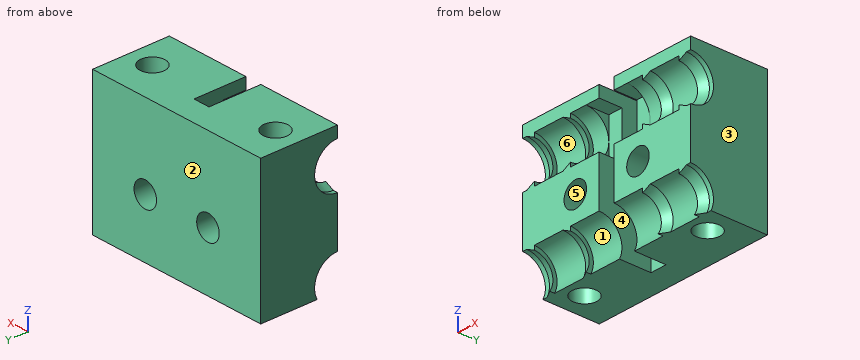
from build123d import *

# Parameters (mm, degrees)
REVOLVE1_ANGLE           = 180
BOSS_EXTRUDE1_DEPTH      = 9.25
BOSS_EXTRUDE1_DEPTH_BACK = 9.25
BOSS_EXTRUDE2_START      = 3.5
BOSS_EXTRUDE2_DEPTH      = 5.75
BOSS_EXTRUDE3_START      = -3.5
BOSS_EXTRUDE3_DEPTH      = 5.75
SKETCH14_W               = 2.5
SKETCH14_H               = 5
CUT_EXTRUDE10_DEPTH      = 13.7
SKETCH13_W               = 5.5
SKETCH13_H               = 2.75
CUT_EXTRUDE9_DEPTH       = 1.75
SKETCH15_W               = 12.7
SKETCH15_H               = 8
CUT_EXTRUDE11_DEPTH      = 6
SKETCH16_W               = 5.122625222
SKETCH16_H               = 5
CUT_EXTRUDE12_DEPTH      = 13.7
SKETCH22_W               = 2.5
SKETCH22_H               = 5
CUT_EXTRUDE17_DEPTH      = 17.877374778
SKETCH17_W               = 10.2
SKETCH17_H               = 16.877374778
BOSS_EXTRUDE4_DEPTH      = 4.25
SKETCH18_R               = 1.5
CUT_EXTRUDE13_DEPTH      = 10.25
SKETCH19_R               = 1.5
CUT_EXTRUDE14_DEPTH      = 6
SKETCH20_R               = 1.5
CUT_EXTRUDE16_DEPTH      = 17.877374778
SKETCH23_W               = 16.877374778
SKETCH23_H               = 3
BOSS_EXTRUDE5_DEPTH      = 1


with BuildPart() as part:
    # Sketch6 → Revolve1 (revolve)
    with BuildSketch(Plane(origin=(0, 0, 0), x_dir=(1, 0, 0), z_dir=(0, 1, 0))):
        Polygon((0, 5), (0, 2.75), (3.81, 2.75), (3.81, 2.242), (4.826, 2.75), (8.636, 2.75), (8.636, 2.242), (9.652, 2.75), (12.7, 2.75), (12.7, 5), align=None)
    revolve(axis=Axis((0, 0, 0), (1, 0, 0)), revolution_arc=REVOLVE1_ANGLE)

    # Sketch9 → Boss-Extrude1 (add, two sides)
    with BuildSketch(Plane.XY) as boss_extrude1_sk:
        Polygon((0, 3.25), (0, 5), (12.7, 5), (12.7, 2.75), align=None)
    extrude(amount=BOSS_EXTRUDE1_DEPTH)
    extrude(boss_extrude1_sk.sketch, amount=-BOSS_EXTRUDE1_DEPTH_BACK)

    # Sketch9_3 → Boss-Extrude2 (add)
    with BuildSketch(Plane.XY.offset(BOSS_EXTRUDE2_START)):
        Polygon((0, 3.25), (12.7, 2.75), (12.7, 0), (0, 0), align=None)
    extrude(amount=BOSS_EXTRUDE2_DEPTH)

    # Sketch9_4 → Boss-Extrude3 (add)
    with BuildSketch(Plane.XY.offset(BOSS_EXTRUDE3_START)):
        Polygon((0, 3.25), (12.7, 2.75), (12.7, 0), (0, 0), align=None)
    extrude(amount=-BOSS_EXTRUDE3_DEPTH)

    # Sketch14 → Cut-Extrude10 (cut, through all)
    with BuildSketch(Plane.ZY):
        with Locations((-8, 2.5)):
            Rectangle(SKETCH14_W, SKETCH14_H)
    extrude(amount=-CUT_EXTRUDE10_DEPTH, mode=Mode.SUBTRACT)

    # Mirror4: part across plane


with BuildPart() as part_1:
    add(part.part)
    add(part.part.mirror(Plane.XY.offset(-5.75)))

    # Sketch13 → Cut-Extrude9 (cut)
    with BuildSketch(Plane.ZY):
        with Locations((0, 1.375)):
            Rectangle(SKETCH13_W, SKETCH13_H)
    extrude(amount=-CUT_EXTRUDE9_DEPTH, mode=Mode.SUBTRACT)

    # Sketch15 → Cut-Extrude11 (cut, through all)
    with BuildSketch(Plane(origin=(0, 5, 0), x_dir=(1, 0, 0), z_dir=(0, 1, 0))):
        with Locations((6.35, 16.75)):
            Rectangle(SKETCH15_W, SKETCH15_H)
    extrude(amount=-CUT_EXTRUDE11_DEPTH, mode=Mode.SUBTRACT)

    # Sketch16 → Cut-Extrude12 (cut, through all)
    with BuildSketch(Plane.ZY):
        with Locations((6.688687389, 2.5)):
            Rectangle(SKETCH16_W, SKETCH16_H)
    extrude(amount=-CUT_EXTRUDE12_DEPTH, mode=Mode.SUBTRACT)

    # Sketch22 → Cut-Extrude17 (cut, through all)
    with BuildSketch(Plane.XY.offset(4.127374778)):
        with Locations((11.45, 2.5)):
            Rectangle(SKETCH22_W, SKETCH22_H)
    extrude(amount=-CUT_EXTRUDE17_DEPTH, mode=Mode.SUBTRACT)


with BuildPart() as body_2:
    # Mirror8: mirrored copy
    add(part_1.part.mirror(Plane.XY.offset(5.397374778)))

    # Sketch19 → Cut-Extrude14 (cut, through all)
    with BuildSketch(Plane(origin=(0, 5, 0), x_dir=(1, 0, 0), z_dir=(0, 1, 0))):
        with Locations((3.175, -16.573374778)):
            Circle(SKETCH19_R)
    extrude(amount=-CUT_EXTRUDE14_DEPTH, mode=Mode.SUBTRACT)


with BuildPart() as part_2:
    add(part_1.part)

    # Sketch17 → Boss-Extrude4 (add)
    with BuildSketch(Plane(origin=(0, 5, 0), x_dir=(1, 0, 0), z_dir=(0, 1, 0))):
        with Locations((5.1, 4.311312611)):
            Rectangle(SKETCH17_W, SKETCH17_H)
    extrude(amount=BOSS_EXTRUDE4_DEPTH)

    # Sketch18 → Cut-Extrude13 (cut, through all)
    with BuildSketch(Plane(origin=(0, 9.25, 0), x_dir=(1, 0, 0), z_dir=(0, 1, 0))):
        with Locations((3.175, 5.778625222)):
            Circle(SKETCH18_R)
    extrude(amount=-CUT_EXTRUDE13_DEPTH, mode=Mode.SUBTRACT)

    # Sketch20 → Cut-Extrude16 (cut, through all)
    with BuildSketch(Plane.XY.offset(4.127374778)):
        with Locations((7.2, 4.75)):
            Circle(SKETCH20_R)
    extrude(amount=-CUT_EXTRUDE16_DEPTH, mode=Mode.SUBTRACT)

    # Sketch23 → Boss-Extrude5 (add)
    with BuildSketch(Plane.ZY):
        with Locations((-4.311312611, 7.75)):
            Rectangle(SKETCH23_W, SKETCH23_H)
    extrude(amount=BOSS_EXTRUDE5_DEPTH)


with BuildPart() as body_3:
    # Mirror9: mirrored copy
    add(part_2.part.mirror(Plane.ZY.offset(1)))

    # Combine1: union part
    add(part_2.part)


solid = body_3.part
The listing builds one solid part. Answer for the finished solid, in the listing's coordinates (mm). Face numbers are marked on the shaded views. A direction names the side the tool comes from. Round coordinates to 2 decimals unless told otherwise and drop trailing zeros. Write each loop counter-clockwise with the first axis right and the second up, starting at its lowest first coordinate (ties: lowest second). Pieces come first, ordered by that corner, then holes. Notation, with made-up numbers: (-26.75, 16.25) - (-3.75, 16.25) arc R18 cw to (-3.75, 26.25) - close; hole circle Ø2 at (-16, 55.5). An arc over 180 degrees is marked (long way). Use a Markdown table: item, result. Add a question column.
1. The part is cut by section A-A (y = 4.75). Write down the section's boundary in (x, z) (3 decimals).
2. A tool of negligible diameter and unlimited length cuts with its end or side. For the marked faces 4, 5 and 6, from which of +Z, -Z, +X, -X, +Y, -Y can it reach the whole face along a straight path? Write none if from no direction.
3. The part is cut by section B-B (z = -3). Write down the section's boundary in (x, y).
4. For a pull along X with two mould halves and no side action, classify the marked faces 1, 2 and 3 as +X half, -X half, draft (parallel to the pull), parting line (faces both ways), or undercut.
5. Consider line 1 (X direction, y = 3, z = -6.25); line 2 (Z direction, x = 2.25, y = 1.5); line 3 (X direction, y = 2, z = -4.75). Determine where each line is inside the solid, lowest interval first.
6. Flat-ended cylindrical pins translate along their axes: P1, Ø3, axis at y = 1, z = -10, coming from the +X side; P2, Ø1.9, axis at x = 1, z = 0, coming from the -Y side; P3, Ø1.9, axis at x = -3, z = 0.5, coming from the -Y side; P4, Ø2, axis at y = 1.5, z = 0.5, coming from the -X side. Find the tip coordinate at first contact, or state that the pin passes through.
7. The part is cut by section D-D (y = 7.75). Write down the section's boundary in (x, z) (3 decimals), and give its area (3 significant figures).
8. The part is cut by section C-C (x = -4). Write down the section's boundary in (y, z), and give its area (3 significant figures).
Reported:
| question | item | result |
|---|---|---|
| 1 | outline | (-12.2, -12.75) - (-10.7, -12.75) - (-10.7, 4.127) - (-12.2, 4.127) - close; (-7.7, -12.75) - (-2, -12.75) - (-2, 4.127) - (-7.7, 4.127) - close; (0, -12.75) - (5.7, -12.75) - (5.7, 4.127) - (0, 4.127) - close; (8.7, -12.75) - (10.2, -12.75) - (10.2, 4.127) - (8.7, 4.127) - close; hole circle Ø3 at (-5.175, -5.779); hole circle Ø3 at (3.175, -5.779) |
| 2 | face 4 | +Z, -Z, -Y |
| 2 | face 5 | +Y, -Y |
| 2 | face 6 | -Y |
| 3 | outline | (-12.2, 0) - (-2, 0) - (-2, 6.25) - (0, 6.25) - (0, 0) - (10.2, 0) - (10.2, 9.25) - (-12.2, 9.25) - close; hole circle Ø3 at (-9.2, 4.75); hole circle Ø3 at (7.2, 4.75) |
| 4 | face 1 | undercut |
| 4 | face 2 | draft |
| 4 | face 3 | +X half |
| 5 | line 1 | -12.2 to -6.6, -3.75 to -2, 0 to 1.75, 4.6 to 10.2 |
| 5 | line 2 | -9.2 to -6.96, -4.6 to -2.3, 2.3 to 4.13 |
| 5 | line 3 | -12.2 to -6.27, -4.08 to -2, 0 to 2.08, 4.27 to 10.2 |
| 6 | P1 | x = 10.2 |
| 6 | P2 | y = 2.69 |
| 6 | P3 | y = 2.53 |
| 6 | P4 | x = -11.31 |
| 7 | outline | (-12.2, -12.75) - (10.2, -12.75) - (10.2, 4.127) - (-12.2, 4.127) - close; hole circle Ø3 at (-5.175, -5.779); hole circle Ø3 at (3.175, -5.779) |
| 7 | area | 364 mm^2 |
| 8 | outline | (0, -8.75) arc R2.75 cw to (2.45, -12.75) - (9.25, -12.75) - (9.25, -6.71) - (0, -6.71) - close; (0, -4.85) - (9.25, -4.85) - (9.25, 4.13) - (0, 4.13) - (0, 2.75) arc R2.75 cw to (0, -2.75) - close |
| 8 | area | 118 mm^2 |
